Autodesk Inventor part; units mm, degrees
ref_plane "YZ Plane" through (0, 0, 0) normal (1, 0, 0) x (0, 1, 0)
ref_plane "XZ Plane" through (0, 0, 0) normal (0, 1, 0) x (-1, 0, 0)
ref_plane "XY Plane" through (0, 0, 0) normal (0, 0, 1) x (1, 0, 0)
sketch "Sketch1" plane through (0, 0, 0) normal (0, 0, 1) x (1, 0, 0)
  line L0 (-35.6004, 16.8538) -> (21.5496, 16.8538)
  line L1 (21.5496, 16.8538) -> (21.5496, -21.2462)
  line L2 (21.5496, -21.2462) -> (-35.6004, -21.2462)
  line L3 (-35.6004, -21.2462) -> (-35.6004, 16.8538)
  point P0 (0, 0)
  dimension "d0" = 57.15
  dimension "d1" = 38.1
extrude "Extrusion1" add sketch "Sketch1" along normal blind 31.75
sketch "Sketch2" plane through (21.5496, -21.2462, 0) normal (1, 0, 0) x (0, 0, -1)
  line L0 (0, 0) -> (0, 38.1)
  line L1 (0, 38.1) -> (-12.7, 38.1)
  line L2 (-12.7, 38.1) -> (-12.7, 12.7)
  line L3 (-12.7, 12.7) -> (0, 12.7)
  line L4 (0, 12.7) -> (0, 38.1)
  point P0 (0, 21.2462)
  dimension "d4" = 25.4
  dimension "d5" = 12.7
extrude "Extrusion2" cut sketch "Sketch2" against normal blind 6.35
sketch "Sketch3" plane through (-35.6004, 16.8538, 31.75) normal (0, 1, 0) x (1, 0, 0)
  line L0 (57.15, 31.75) -> (57.15, 0)
  line L1 (57.15, 0) -> (31.75, 0)
  line L2 (31.75, 0) -> (31.75, 19.05)
  line L3 (31.75, 19.05) -> (57.15, 19.05)
  line L4 (57.15, 19.05) -> (57.15, 0)
  point P0 (35.6004, 31.75)
  dimension "d8" = 19.05
  dimension "d9" = 25.4
extrude "Extrusion3" cut sketch "Sketch3" against normal blind 25.4
sketch "Sketch4" plane through (0, 0, 31.75) normal (0, 0, 1) x (1, 0, 0)
  line L0 (-35.6004, -21.2462) -> (-16.5504, -21.2462)
  line L1 (-16.5504, -21.2462) -> (-16.5504, 4.1538)
  line L2 (-16.5504, 4.1538) -> (-35.6004, 4.1538)
  line L3 (-35.6004, 4.1538) -> (-35.6004, -21.2462)
  point P0 (0, 0)
  dimension "d12" = 19.05
  dimension "d13" = 25.4
extrude "Extrusion4" cut sketch "Sketch4" against normal blind 50.8
properties part number "Figure 7_27_8"
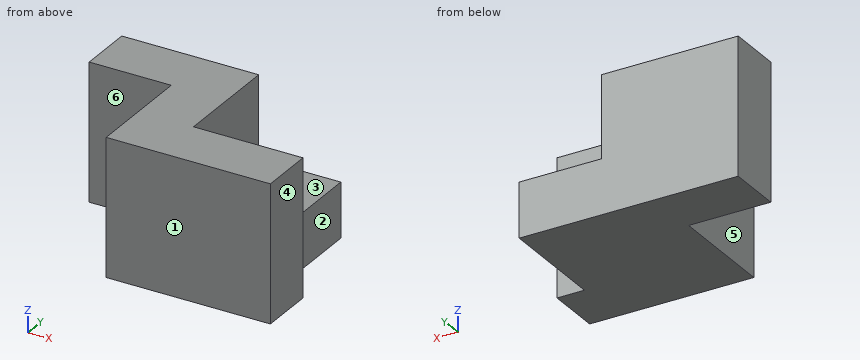
Source: CAD feature listing. Evaluate the final solid. Frame: model axes, mm. Face numbers are marked on the shaded views. A direction names the side the tool comes from. Round coordinates to 2 decimals unless told otherwise and drop trailing zeros. Loops run counter-clockwise (first coordinate to the right, second up) from the corner with the lowest first, then second, coordinate; pieces in that order, holes last. Notation, with made-up numbers: (-20, 12) -> (10, 12) arc R13 cw to (10, 26) -> close; hole circle Ø10 at (9.25, 69.5). An arc over 180 degrees is marked (long way). Answer as a JSON object with one key per item and string values. Group by question number.
Q1. Section query D-D (z = 16). Output: boundary loops of the cut face in (x, y).
Q2. Section query A-A (z = 6). Output: boundary loops of the cut face in (x, y), plus the area to 3 significant figures.
Q3. Section query B-B (x = 6). Output: boundary loops of the cut face in (y, z).
Q4. Contact query for flat-ended pins moving along their axis: P1, Ø5.5, axis at x = -22.5, z = 21, coming from the -Y side; P2, Ø10, axis at y = 5.5, z = 5, coming from the +X side; P3, Ø2, axis at x = -1.5, y = -2.5, coming from the +Z side. Output: stop coordinate, or through.
Q5. Access query for the marked faces 1, 2 and 3. Directions: +Z, -Z, +X, -X, +Y, -Y. A direction counts if a zero-diameter tool reaches every point of the face in a straight line with its end or side. Return the directions, or none.
Q6. Mould query, pull axis X, two halves, no side actions, for the marked faces 4, 5 and 6. Classes: pulls with the +X half, pulls with the -X half, needs draft (parallel to the pull), parting line crosses it, or undercut.
Q7. Section query C-C (y = 9). Output: boundary loops of the cut face in (x, z), plus the area to 3 significant figures.
Q8. Ray query, line 1 (Y direction, x = -23, z = 21); line 2 (X direction, y = 11, z = 26.5); line 3 (Z direction, x = 10.5, y = 4). Return the intervals inside material, ascending. Write a range as from..to.
Completed:
{
 "1": {"outline": "(-35.6, 4.15) -> (-16.55, 4.15) -> (-16.55, -21.25) -> (21.55, -21.25) -> (21.55, -8.55) -> (-3.85, -8.55) -> (-3.85, 16.85) -> (-35.6, 16.85) -> close"},
 "2": {"outline": "(-35.6, 4.15) -> (-16.55, 4.15) -> (-16.55, -21.25) -> (21.55, -21.25) -> (21.55, -8.55) -> (15.2, -8.55) -> (15.2, 16.85) -> (-35.6, 16.85) -> close", "area": "1,530 mm²"},
 "3": {"outline": "(-21.25, 0) -> (16.85, 0) -> (16.85, 12.7) -> (-8.55, 12.7) -> (-8.55, 31.75) -> (-21.25, 31.75) -> close"},
 "4": {"P1": "y = 4.15", "P2": "x = 15.2", "P3": "z = 12.7"},
 "5": {"face 1": "+Z, -Z, +X, -X, -Y", "face 2": "+Z, -Z, +X, +Y", "face 3": "+Z, +X, +Y"},
 "6": {"face 4": "pulls with the +X half", "face 5": "pulls with the -X half", "face 6": "needs draft"},
 "7": {"outline": "(-35.6, 0) -> (15.2, 0) -> (15.2, 12.7) -> (-3.85, 12.7) -> (-3.85, 31.75) -> (-35.6, 31.75) -> close", "area": "1,250 mm²"},
 "8": {"line 1": "4.15..16.85", "line 2": "-35.6..-3.85", "line 3": "0..12.7"}
}
